Design review of the part shown in the three views and the two pictorial views. Dimensions are in mm from the part's minimum x, y and z. Round coordinates to 2 decimals unless told otherwise and drop trailing zeros. Loops run counter-clockwise (first coordinate to the right, second up) from the corner with the lowest first, then second, coordinate; pieces in that order, holes last. Notation, with made-up numbers: (-33, 8) -> (-11, 8) arc R15 cw to (-11, 22) -> close; hole circle Ø8 at (-29.75, 39). An arc over 180 degrees is marked (long way). Use a Markdown table: item, result. Add a question column.
1) Consider section A-A on z = 50.8. Give the boundary of the cut face in (x, y), plus the area to 3 significant figures.
2) Wall thickness on probe 1 along X at (y, z) = (9.75, 50.8); probe 2 along X at (y, z) = (2, 60.5) (1 decimal); probe 3 along Z at (x, y) = (110, 8): over which ranges is each line inside the solid? List them lowest first.
3) Consider section B-B on z = 100.5. Give the boundary of the cut face in (x, y), plus the area to 3 significant figures.
4) Consider section D-D on y = 2.25. Give the boundary of the cut face in (x, z) (1 decimal), plus the area to 3 significant figures.
5) Consider section C-C on x = 117. Give the boundary of the cut face in (y, z).
6) Insertion check: pin 1 (4 mm diameter, centred on x = 158.5, y = 8.5, fed in from +Z). The pin has a flat end and moves straight along its axis. Give the tip position at first contact, or say it passes through.
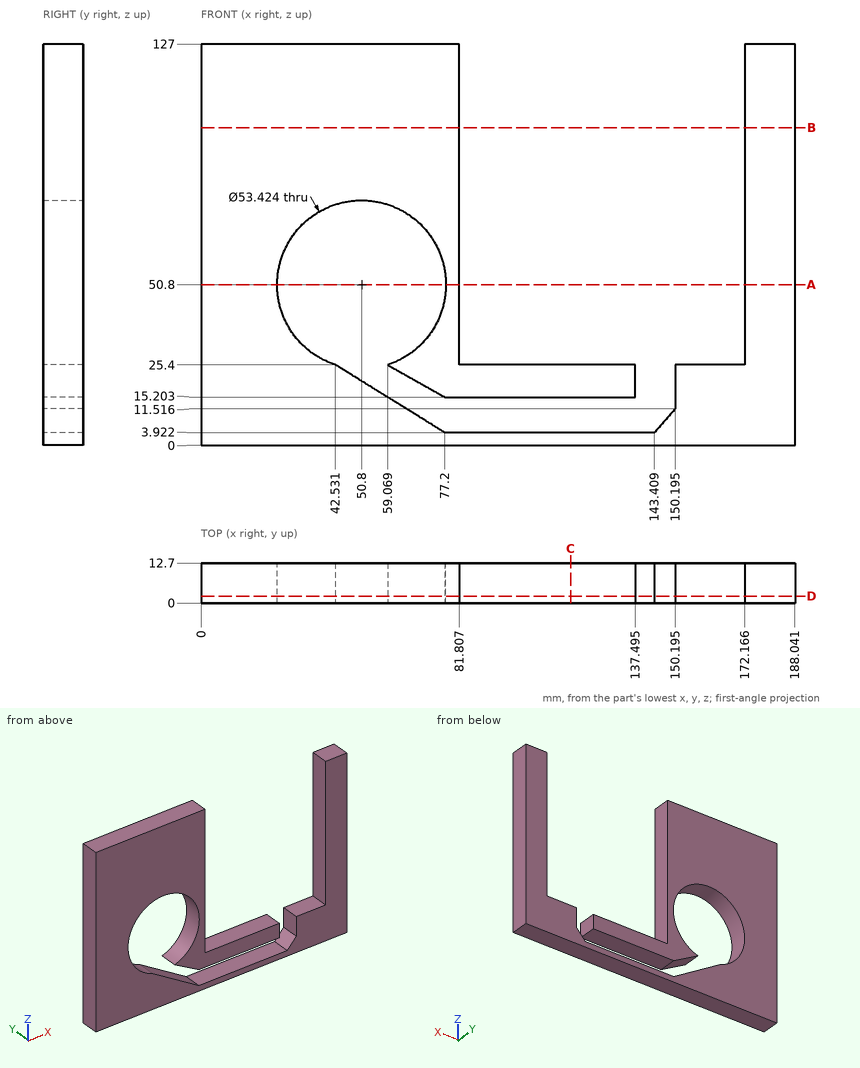
Result set:
| question | item | result |
|---|---|---|
| 1 | outline | (0, 0) -> (24.09, 0) -> (24.09, 12.7) -> (0, 12.7) -> close; (77.51, 0) -> (81.81, 0) -> (81.81, 12.7) -> (77.51, 12.7) -> close; (172.17, 0) -> (188.04, 0) -> (188.04, 12.7) -> (172.17, 12.7) -> close |
| 1 | area | 562 mm2 |
| 2 | probe 1 | 0 to 24.09, 77.51 to 81.81, 172.17 to 188.04 |
| 2 | probe 2 | 0 to 25.9, 75.7 to 81.8, 172.2 to 188 |
| 2 | probe 3 | 0 to 3.92, 15.2 to 25.4 |
| 3 | outline | (0, 0) -> (81.81, 0) -> (81.81, 12.7) -> (0, 12.7) -> close; (172.17, 0) -> (188.04, 0) -> (188.04, 12.7) -> (172.17, 12.7) -> close |
| 3 | area | 1,240 mm2 |
| 4 | outline | (0, 0) -> (188, 0) -> (188, 127) -> (172.2, 127) -> (172.2, 25.4) -> (150.2, 25.4) -> (150.2, 11.5) -> (143.4, 3.9) -> (77.2, 3.9) -> (42.5, 25.4) arc R26.7 cw (long way) to (59.1, 25.4) -> (77.2, 15.2) -> (137.5, 15.2) -> (137.5, 25.4) -> (81.8, 25.4) -> (81.8, 127) -> (0, 127) -> close |
| 4 | area | 11,300 mm2 |
| 5 | outline | (0, 0) -> (12.7, 0) -> (12.7, 3.92) -> (0, 3.92) -> close; (0, 15.2) -> (12.7, 15.2) -> (12.7, 25.4) -> (0, 25.4) -> close |
| 6 | pin 1 | z = 25.4 |
